from build123d import *

# Parameters (mm, degrees)
EXTRUDE_1_DEPTH     = 74.5
CUT_EXTRUDE_1_DEPTH = 4
CUT_EXTRUDE_2_DEPTH = 4
CUT_EXTRUDE_3_DEPTH = 62
CUT_EXTRUDE_4_REACH = 124.795
SKETCH_5_W          = 45.7
SKETCH_5_H          = 21.3
SKETCH_6_R          = 0.998844791
SKETCH_6_R_2        = 1.4
EXTRUDE_2_DEPTH     = 3
CUT_EXTRUDE_5_REACH = 124.795
SKETCH_7_W          = 10.739655284
SKETCH_7_H          = 11.312103995
EXTRUDE_3_DEPTH     = 57.007858917
CUT_EXTRUDE_6_DEPTH = 74.5


with BuildPart() as part:
    # 草圖1 → 填料-伸長1 (new body)
    with BuildSketch(Plane.XY):
        Polygon((-93.525975622, -88.048741595), (-102.106102641, -83.095002951), (-103.606102641, -85.693079162), (-97.519536964, -89.207159494), (-39.813710348, -122.523634025), (36.141513372, -78.670865164), (40.257538776, -76.294476789), (36.757538776, -74.273750847), (34.391513372, -75.639776251), (-1.383477376, -51.675674636), (-30.525975622, -51.675674636), align=None)
    extrude(amount=EXTRUDE_1_DEPTH)

    # 草圖2 → 除料-伸長1 (cut)
    with BuildSketch(Plane(origin=(0, 0, 0), x_dir=(-1, 0, 0), z_dir=(0, 0, -1))):
        Polygon((-40.257538776, -76.294476789), (-36.757538776, -74.273750847), (-34.391513372, -75.639776251), (-37.891513372, -77.660502193), align=None)
        Polygon((102.106102641, -83.095002951), (93.525975622, -88.048741595), (96.525975622, -89.780792402), (103.606102641, -85.693079162), align=None)
    extrude(amount=-CUT_EXTRUDE_1_DEPTH, mode=Mode.SUBTRACT)

    # 草圖3 → 除料-伸長2 (cut)
    with BuildSketch(Plane(origin=(0, 0, 0), x_dir=(-1, 0, 0), z_dir=(0, 0, -1))):
        Polygon((-33.635403301, -80.117768489), (-31.970986825, -74.018371384), (-37.891513372, -77.660502193), align=None)
    extrude(amount=-CUT_EXTRUDE_2_DEPTH, mode=Mode.SUBTRACT)

    # 草圖4 → 除料-伸長3 (cut)
    with BuildSketch(Plane.XY.offset(74.5)):
        Polygon((-60.217268861, -110.743634025), (-31.713339402, -61.373379987), (12.19414857, -86.723379987), (7.19414857, -95.383634025), (-39.813710348, -122.523634025), align=None)
    extrude(amount=-CUT_EXTRUDE_3_DEPTH, mode=Mode.SUBTRACT)

    # 草圖5 → 除料-伸長4 (cut, up to next)
    with BuildSketch(Plane(origin=(-34.503787943, -59.762313771, 0), x_dir=(0.8660254037844352, -0.500000000000006, 0), z_dir=(-0.500000000000006, -0.8660254037844352, 0)), mode=Mode.PRIVATE) as cut_extrude_4_sk1:
        with Locations((27.672132433, 23.15)):
            Rectangle(SKETCH_5_W, SKETCH_5_H)
    cut_extrude_4_tool1 = extrude(cut_extrude_4_sk1.sketch, amount=-CUT_EXTRUDE_4_REACH, mode=Mode.PRIVATE) & part.part
    add(cut_extrude_4_tool1.solids().sort_by_distance((-10.539018, -73.59838, 23.15))[0], mode=Mode.SUBTRACT)

    # 草圖6 → 填料-伸長2 (add)
    # profile 1 of 2: a face of its own
    with BuildSketch(Plane(origin=(-34.503787943, -59.762313771, 0), x_dir=(0.8660254037844352, -0.500000000000006, 0), z_dir=(-0.500000000000006, -0.8660254037844352, 0))):
        with BuildLine():
            Line((4.822132433, 17.5), (4.822132433, 12.5))
            Line((4.822132433, 12.5), (9.822132433, 12.5))
            Line((9.822132433, 12.5), (9.822132433, 16))
            ThreePointArc((9.822132433, 16), (9.382792604, 17.060660172), (8.322132433, 17.5))
            Line((8.322132433, 17.5), (4.822132433, 17.5))
        make_face()
        with Locations((7.322132433, 15)):
            Circle(SKETCH_6_R, mode=Mode.SUBTRACT)
    # profile 2 of 2: a face of its own
    with BuildSketch(Plane(origin=(-34.503787943, -59.762313771, 0), x_dir=(0.8660254037844352, -0.500000000000006, 0), z_dir=(-0.500000000000006, -0.8660254037844352, 0))):
        with BuildLine():
            Line((50.522132433, 28.8), (50.522132433, 33.8))
            Line((50.522132433, 33.8), (45.522132433, 33.8))
            Line((45.522132433, 33.8), (45.522132433, 30.299999983))
            ThreePointArc((45.522132433, 30.299999983), (45.961472267, 29.239339822), (47.022132433, 28.8))
            Line((47.022132433, 28.8), (50.522132433, 28.8))
        make_face()
        with Locations((48.022132433, 31.3)):
            Circle(SKETCH_6_R_2, mode=Mode.SUBTRACT)
    extrude(amount=-EXTRUDE_2_DEPTH)

    # 草圖7 → 除料-伸長5 (cut, up to next)
    with BuildSketch(Plane(origin=(-34.503787943, -59.762313771, 0), x_dir=(0.8660254037844352, -0.500000000000006, 0), z_dir=(-0.500000000000006, -0.8660254037844352, 0)), mode=Mode.PRIVATE) as cut_extrude_5_sk1:
        with Locations((27.54107715, 46.72819857)):
            Rectangle(SKETCH_7_W, SKETCH_7_H)
    cut_extrude_5_tool1 = extrude(cut_extrude_5_sk1.sketch, amount=-CUT_EXTRUDE_5_REACH, mode=Mode.PRIVATE) & part.part
    add(cut_extrude_5_tool1.solids().sort_by_distance((-10.652515, -73.532852, 46.728199))[0], mode=Mode.SUBTRACT)

    # 草圖8 → 填料-伸長3 (add)
    with BuildSketch(Plane(origin=(-34.503787943, -59.762313771, 0), x_dir=(0.8660254037844352, -0.500000000000006, 0), z_dir=(-0.500000000000006, -0.8660254037844352, 0))):
        Polygon((22.171249508, 41.072146572), (22.171249508, 52.384250567), (32.910904792, 52.384250567), (32.910904792, 41.072146572), (53.922132433, 41.072146572), (53.922132433, 74.5), (3.222132433, 74.5), (3.222132433, 41.072146572), align=None)
    extrude(amount=EXTRUDE_3_DEPTH)

    # 草圖9 → 除料-伸長6 (cut)
    with BuildSketch(Plane(origin=(0, 0, 0), x_dir=(-1, 0, 0), z_dir=(0, 0, -1))):
        Polygon((39.813710348, -122.523634025), (16.309780889, -136.093634025), (-7.19414857, -95.383634025), align=None)
    extrude(amount=-CUT_EXTRUDE_6_DEPTH, mode=Mode.SUBTRACT)


solid = part.part
Work out the finished part from the listing and answer in its coordinate system (mm). A direction names the side the tool comes from. Give positions to 0.01 mm unless a question says otherwise; leave off trailing zeros. Write each loop counter-clockwise with the first axis right and the second up, starting at its lowest first coordinate (ties: lowest second). Pieces come first, ordered by that corner, then holes. Notation, with made-up numbers: M -6,83.5 L 24,83.5 A19 cw 24,100.5 Z; hole C 82.5,19 d11. An arc over 180 degrees is marked long. Answer as CSV lines item,"result".
Q1. Find the intervals of material crossed by probe 1 along Z at (x, y) = (-7.5, -66.5); probe 2 along Z at (x, y) = (-49, -97.5); probe 3 along Y at (x, z) = (-17, 43.5), in increasing order. Write a range as [from, to].
A:
probe 1,"z = [0, 12.5], [33.8, 41.07], [52.38, 74.5]"
probe 2,"z = [0, 12.5], [41.07, 74.5]"
probe 3,"y = [-109.35, -95.27], [-73.79, -51.68]"
Q2. A cutting plane is placed at B-B on y = -58. Write down the section's boundary in (x, z).
A:
outline,"M -41.48,0 L 8.06,0 L 8.06,12.5 L -27.92,12.5 L -27.92,33.8 L 8.06,33.8 L 8.06,74.5 L -41.48,74.5 Z; hole M -7.89,41.07 L 4.52,41.07 L 4.52,52.38 L -7.89,52.38 Z"
Q3. A cutting plane is placed at D-D on z = 64. Write down the section's boundary in (x, y) (3 decimals).
A:
outline,"M -103.606,-85.693 L -39.814,-122.524 L 40.258,-76.294 L 36.758,-74.274 L 34.392,-75.64 L -1.383,-51.676 L -30.526,-51.676 L -93.526,-88.049 L -102.106,-83.095 Z"
Q4. A tool of negligible diameter and unlimited length cuts with its end or side. For faces 5 (the flat face through (-5, -63, 41.072)), 6 (the flat face through (-98, -86, 4)), 7 (the cylindrical face through (6.03, -81.46, 29.25)), from which of +Z, -Z, +X, -X, +Y, -Y can it reach the whole face along a straight path? Write none if from no direction.
A:
face 5,"none"
face 6,"-Z, -X, +Y"
face 7,"+Y"
Q5. The mould has two halves that part along Y. Classify faces 1 (the flat face through (14.632, -75.7, 23.001)), 2 (the flat face through (-23.743, -85.467, 46.649)), 3 (the flat face through (-27.34, -57, 23)), 4 (the flat face through (-31, -81, 74.5)): +Y half, -Y half, draft (parallel to the pull), parting line (faces both ways), or undercut.
A:
face 1,"+Y half"
face 2,"undercut"
face 3,"undercut"
face 4,"draft"
Q6. A cutting plane is placed at C-C on x = -20.5. Write down the section's boundary in (y, z), plus the area to 3 significant figures.
A:
outline,"M -111.37,0 L -51.68,0 L -51.68,12.5 L -111.37,12.5 Z; M -111.37,41.07 L -101.33,41.07 L -101.33,52.38 L -79.85,52.38 L -79.85,41.07 L -67.85,41.07 L -67.85,33.8 L -51.68,33.8 L -51.68,74.5 L -111.37,74.5 Z"
area,"2,620 mm²"
Q7. A cutting plane is placed at A-A on z = 43. Write down the section's boundary in (x, y) (3 decimals).
A:
outline,"M -103.606,-85.693 L -43.807,-120.218 L -4.234,-51.676 L -30.526,-51.676 L -93.526,-88.049 L -102.106,-83.095 Z; M -29.198,-116.395 L 40.258,-76.294 L 36.758,-74.274 L 34.392,-75.64 L 5.504,-56.289 Z"
Q8. Given P1, Ø3, axis at x = -59, z = 31, coming from the -Y side; P2, Ø5, axis at y = -72.5, z = 32.5, coming from the -X side; P3, Ø8, axis at y = -96, z = 18.5, coming from the +X side, each flat-ended and moving along its own axis, determine where each tip first touches the part or whether it passes through.
A:
P1,"stops at y = -110.74"
P2,"stops at x = -70.92"
P3,"stops at x = 13.05"
